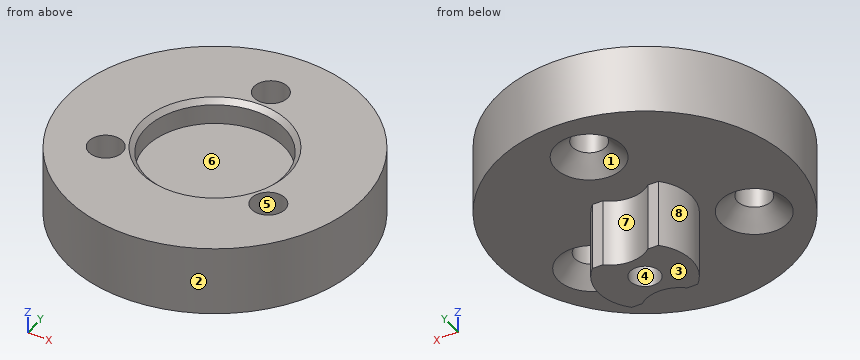
from build123d import *

# Parameters (mm, degrees)
SKETCH_R        = 15
SKETCH_R_2      = 1.7
PAD_DEPTH       = 7
PAD001_DEPTH    = 6.9
SKETCH006_R     = 3.5
POCKET003_DEPTH = 6.9
SKETCH003_R     = 1.5
POCKET004_DEPTH = 7.3
SKETCH008_R     = 7
POCKET_DEPTH    = 2.5
CHAMFER_SIZE    = 1.7
CHAMFER001_SIZE = 1.7
CHAMFER002_SIZE = 1.7
CHAMFER003_SIZE = 0.5


with BuildPart() as part:
    # Sketch → Pad (new body)
    with BuildSketch(Plane.XY):
        Circle(SKETCH_R)
        with Locations((0, 9.526279)):
            Circle(SKETCH_R_2, mode=Mode.SUBTRACT)
        with Locations((-8.25, -4.76314)):
            Circle(SKETCH_R_2, mode=Mode.SUBTRACT)
        with Locations((8.25, -4.76314)):
            Circle(SKETCH_R_2, mode=Mode.SUBTRACT)
    extrude(amount=PAD_DEPTH)

    # Sketch004 → Pad001 (new body)
    with BuildSketch(Plane(origin=(0, 0, 0), x_dir=(1, 0, 0), z_dir=(0, 0, -1))):
        with BuildLine():
            Line((-3.35, 3.35), (3.35, 3.35))
            ThreePointArc((3.35, -3.35), (4.737615, 0), (3.35, 3.35))
            Line((3.35, -3.35), (-3.35, -3.35))
            ThreePointArc((-3.35, 3.35), (-4.737615, 0), (-3.35, -3.35))
        make_face()
    extrude(amount=PAD001_DEPTH)

    # Sketch006 → Pocket003 (cut)
    with BuildSketch(Plane(origin=(0, 0, -6.9), x_dir=(1, 0, 0), z_dir=(0, 0, -1))):
        with Locations((0, 6)):
            Circle(SKETCH006_R)
        with Locations((0, -6)):
            Circle(SKETCH006_R)
    extrude(amount=-POCKET003_DEPTH, mode=Mode.SUBTRACT)

    # Sketch003 → Pocket004 (cut)
    with BuildSketch(Plane(origin=(0, 0, -6.9), x_dir=(1, 0, 0), z_dir=(0, 0, -1))):
        Circle(SKETCH003_R)
    extrude(amount=-POCKET004_DEPTH, mode=Mode.SUBTRACT)

    # Sketch008 → Pocket (cut)
    with BuildSketch(Plane.XY.offset(7)):
        Circle(SKETCH008_R)
    extrude(amount=-POCKET_DEPTH, mode=Mode.SUBTRACT)

    # Chamfer
    chamfer_edges = [part.edges().sort_by_distance(p)[0] for p in [
        (-9.95, -4.76314, 0),
    ]]
    chamfer(chamfer_edges, length=CHAMFER_SIZE)

    # Chamfer001
    chamfer001_edges = [part.edges().sort_by_distance(p)[0] for p in [
        (6.55, -4.76314, 0),
    ]]
    chamfer(chamfer001_edges, length=CHAMFER001_SIZE)

    # Chamfer002
    chamfer002_edges = [part.edges().sort_by_distance(p)[0] for p in [
        (-0.219827, 11.212007, 0),
    ]]
    chamfer(chamfer002_edges, length=CHAMFER002_SIZE)

    # Chamfer003
    chamfer003_edges = [part.edges().sort_by_distance(p)[0] for p in [
        (-7, 0, 7),
    ]]
    chamfer(chamfer003_edges, length=CHAMFER003_SIZE)


solid = part.part
Could you check a few things on this model? Use its own coordinates, in mm. Face numbers are marked on the shaded views. A direction names the side the tool comes from. Coordinates: 2 decimals unless noted, no trailing zeros. Write each loop counter-clockwise with the first axis right and the second up, starting at its lowest first coordinate (ties: lowest second). Pieces come first, ordered by that corner, then holes. Notation, with made-up numbers: (72, -39) - (124, -39) arc R15 cw to (124, -25) - close; hole circle Ø9 at (84.25, 17). An arc over 180 degrees is marked (long way). Put each result on its own line as item: value. Start each with the question number.
Q1. I want a section at A-A on z = -4.75. Write out the boundary of the cut face in (x, y).
Q2. Please list where these lines run through material, in increasing order: L1, parallel to Y at x = 0, z = 5.65; L2, parallel to Y at x = 0, z = 3.8; L3, parallel to X at y = -5.75, z = 1.
Q3. I want a section at D-D on x = -8.25. Write out the boundary of the cut face in (y, z).
Q4. Thinking about a two-plate mould opening in Y: for the marked faces 1, 2 and 3, which applies, pulls with the +Y half, pulls with the -Y half, needs draft (parallel to the pull), parting line crosses it, or undercut?
Q5. I want a section at C-C on y = 0. Write out the boundary of the cut face in (x, z).
Q6. Which directions (+Z, -Z, +X, -X, +Y, -Y) give clear straight access to the entire face, cutting with the end or side of a thin tool? Please do the marked faces 4, 5, 6, 7 and 8.
Q7. I'm going to push flat-ended pins straight in: P1, Ø0.9, axis at x = 2.5, z = -4, coming from the +Y side; P2, Ø7, axis at x = 0, y = 2, coming from the +Z side; P3, Ø4, axis at y = 5, z = 1, coming from the -X side; P4, Ø2, axis at x = 8.25, y = -4.76, coming from the +Z side. Where does each tip first touch, or does it pass through?
Q8. I want a section at B-B on x = 0. Write out the boundary of the cut face in (y, z).
Checks:
1. outline: (-3.35, -3.35) - (-2.29, -3.35) arc R3.5 cw to (2.29, -3.35) - (3.35, -3.35) arc R4.74 ccw to (3.35, 3.35) - (2.29, 3.35) arc R3.5 cw to (-2.29, 3.35) - (-3.35, 3.35) arc R4.74 ccw to start; hole circle Ø3 at (0, 0)
2. L1: -15 to -7, 7 to 7.83, 11.23 to 15
2. L2: -15 to 7.83, 11.23 to 15
2. L3: -13.85 to -10.44, -6.06 to 6.06, 10.44 to 13.85
3. outline: (-12.53, 0) - (-8.16, 0) - (-6.46, 1.7) - (-6.46, 7) - (-12.53, 7) - close; (-3.06, 1.7) - (-1.36, 0) - (12.53, 0) - (12.53, 7) - (-3.06, 7) - close
4. face 1: undercut
4. face 2: parting line crosses it
4. face 3: needs draft
5. outline: (-15, 0) - (-4.74, 0) - (-4.74, -6.9) - (-1.5, -6.9) - (-1.5, 0.4) - (1.5, 0.4) - (1.5, -6.9) - (4.74, -6.9) - (4.74, 0) - (15, 0) - (15, 7) - (7.5, 7) - (7, 6.5) - (7, 4.5) - (-7, 4.5) - (-7, 6.5) - (-7.5, 7) - (-15, 7) - close
6. face 4: -Z
6. face 5: +Z, -Z
6. face 6: +Z
6. face 7: -Z, +Y
6. face 8: -Z, -X
7. P1: y = 3.35
7. P2: z = 4.5
7. P3: x = -14.7
7. P4: through
8. outline: (-15, 0) - (-2.5, 0) - (-2.5, -6.9) - (-1.5, -6.9) - (-1.5, 0.4) - (1.5, 0.4) - (1.5, -6.9) - (2.5, -6.9) - (2.5, 0) - (6.13, 0) - (7.83, 1.7) - (7.83, 7) - (7.5, 7) - (7, 6.5) - (7, 4.5) - (-7, 4.5) - (-7, 6.5) - (-7.5, 7) - (-15, 7) - close; (11.23, 1.7) - (12.93, 0) - (15, 0) - (15, 7) - (11.23, 7) - close
